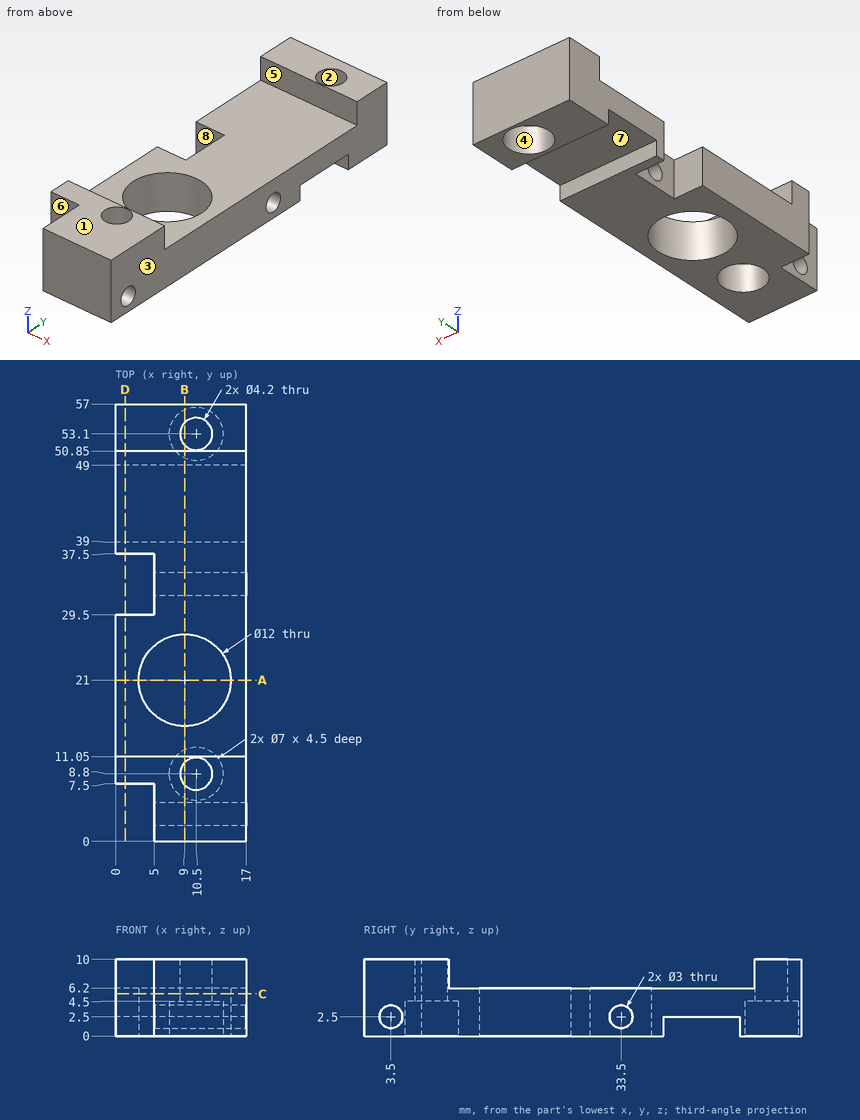
Geometry check sheet. Reference: drawing and pictorial views, mm from the part's lowest x, y, z. A direction names the side the tool comes from. Round coordinates to 2 decimals unless told otherwise and drop trailing zeros. Loops run counter-clockwise (first coordinate to the right, second up) from the corner with the lowest first, then second, coordinate; pieces in that order, holes last. Notation, with made-up numbers: (9, 2.25) - (66, 2.25) arc R11 cw to (66, 14.25) - close; hole circle Ø10 at (53, 56). An arc over 180 degrees is marked (long way). Answer in a Markdown table with one row per item. Add a question column.
Q1. Section check C-C on z = 5.5. Enter the section's corners in (x, y).
Q2. Section check A-A on y = 21. Enter the section's corners in (x, z).
Q3. Section check D-D on x = 1.25. Enter the section's corners in (y, z).
Q4. Tool access check on the marked faces 4, 5, 6, 7 and 8. Record the directions out of +Z, -Z, +X, -X, +Y, -Y that give a thin tool (end or side, any length) a straight path to the whole face; none if there is none.
Q5. Section check B-B on x = 9. State how many separate pieces and enclosed holes the cut face has, plus the area to 3 significant figures.
Q6. Release check for a two-part mould opening along X. For the marked faces 1, 2 and 3 record: pulls with the +X half, pulls with the -X half, needs draft (parallel to the pull), parting line crosses it, or undercut.
Q7. Gauge pin test, flat ends, axial feed: pin 1 (3 mm diameter, centred on x = 7.5, z = 7.5, fed in from -Y); pin 2 (2.5 mm diameter, centred on x = 10.5, y = 53.1, fed in from -Z); pin 3 (2 mm diameter, centred on x = 12, y = 51.5, fed in from -Z); pin 4 (8 mm diameter, centred on x = 7.5, y = 44.5, fed in from -Z). Record the tip position at first contact, or that the pin passes through.
Q8. Material ranges on line 1 (Y direction, x = 10.5, z = 6.9); line 2 (Y direction, x = 4, z = 8); line 3 (Y direction, x = 7.75, z = 8.75), recorded low to high.
Found:
| question | item | result |
|---|---|---|
| 1 | outline | (0, 7.5) - (5, 7.5) - (5, 0) - (17, 0) - (17, 57) - (0, 57) - (0, 37.5) - (5, 37.5) - (5, 29.5) - (0, 29.5) - close; hole circle Ø12 at (9, 21); hole circle Ø4.2 at (10.5, 8.8); hole circle Ø4.2 at (10.5, 53.1) |
| 2 | outline | (0, 0) - (3, 0) - (3, 6.2) - (0, 6.2) - close; (15, 0) - (17, 0) - (17, 6.2) - (15, 6.2) - close |
| 3 | outline | (7.5, 0) - (29.5, 0) - (29.5, 6.2) - (11.05, 6.2) - (11.05, 10) - (7.5, 10) - close; (37.5, 0) - (39, 0) - (39, 2.5) - (49, 2.5) - (49, 0) - (57, 0) - (57, 10) - (50.85, 10) - (50.85, 6.2) - (37.5, 6.2) - close |
| 4 | face 4 | -Z |
| 4 | face 5 | +Z, +X, -X |
| 4 | face 6 | +Z, -Z, -X, -Y |
| 4 | face 7 | -Z, +X, -X |
| 4 | face 8 | +Z, -Z, -X |
| 5 | separate pieces | 4 |
| 5 | enclosed holes | 2 |
| 5 | area | 216 mm² |
| 6 | face 1 | needs draft |
| 6 | face 2 | undercut |
| 6 | face 3 | pulls with the +X half |
| 7 | pin 1 | stops at y = 0 |
| 7 | pin 2 | passes through |
| 7 | pin 3 | stops at z = 4.5 |
| 7 | pin 4 | stops at z = 2.5 |
| 8 | line 1 | y = 0 to 6.7, 10.9 to 11.05, 50.85 to 51, 55.2 to 57 |
| 8 | line 2 | y = 7.5 to 11.05, 50.85 to 57 |
| 8 | line 3 | y = 0 to 11.05, 50.85 to 57 |
